```python
from build123d import *

# Parameters (mm, degrees)
BOSS_EXTRUDE1_DEPTH            = 34
BOSS_EXTRUDE1_2_DEPTH          = 34
SKETCH5_W                      = 38.2
SKETCH5_H                      = 34
BOSS_EXTRUDE2_DEPTH            = 16
BOSS_EXTRUDE7_REACH            = 77.954
SKETCH12_W                     = 2
SKETCH12_H                     = 5
BOSS_EXTRUDE8_REACH            = 79.938
SKETCH13_W                     = 2
SKETCH13_H                     = 5
CUT_EXTRUDE1_START             = 2
SKETCH6_W                      = 4
SKETCH6_H                      = 5
CUT_EXTRUDE1_DEPTH             = 14
SKETCH7_W                      = 49
SKETCH7_H                      = 44
BOSS_EXTRUDE3_DEPTH            = 2
SKETCH8_W                      = 10
SKETCH8_H                      = 5
SKETCH8_W_2                    = 2
BOSS_EXTRUDE5_DEPTH            = 45
CUT_EXTRUDE2_REACH             = 97.297
SKETCH9_W                      = 6
SKETCH9_H                      = 44
CUT_EXTRUDE2_DIRECTION_2_REACH = 97.297
SKETCH10_W                     = 23
SKETCH10_H                     = 24
CUT_EXTRUDE3_DEPTH             = 16
SKETCH11_W                     = 2
SKETCH11_H                     = 5
BOSS_EXTRUDE6_DEPTH            = 37
SKETCH14_W                     = 5
SKETCH14_H                     = 34
CUT_EXTRUDE4_DEPTH             = 5.320889


with BuildPart() as part:
    # Sketch4 → Boss-Extrude1 (new body)
    with BuildSketch(Plane.XY):
        Polygon((0, 0), (-14.095389312, 0), (0, 5.13030215), align=None)
    extrude(amount=BOSS_EXTRUDE1_DEPTH)



with BuildPart() as body_2:
    # Sketch4 → Boss-Extrude1 2 (new body)
    with BuildSketch(Plane.XY):
        Polygon((52.295389312, 0), (38.2, 5.13030215), (38.2, 0), align=None)
    extrude(amount=BOSS_EXTRUDE1_2_DEPTH)


with BuildPart() as part_1:
    add(part.part)

    add(body_2.part)  # Boss-Extrude2 merges body 2
    # Sketch5 → Boss-Extrude2 (add)
    with BuildSketch(Plane(origin=(0, 0, 0), x_dir=(1, 0, 0), z_dir=(0, 1, 0))):
        with Locations((19.1, -17)):
            Rectangle(SKETCH5_W, SKETCH5_H)
    extrude(amount=BOSS_EXTRUDE2_DEPTH)

    # Boss-Extrude7: up to this plane
    boss_extrude7_end = Plane(origin=(0, 16, 0), z_dir=(1, 0, 0))
    # Sketch12 → Boss-Extrude7 (add, up to the surface)
    with BuildSketch(Plane(origin=(-12.446541984, -4.530170802, 0), x_dir=(0, 0, -1), z_dir=(0.9396926207859105, 0.3420201433256627, 0)), mode=Mode.PRIVATE) as boss_extrude7_sk1:
        with Locations((-1, 7.320907073)):
            Rectangle(SKETCH12_W, SKETCH12_H)
    boss_extrude7_tool1 = split(extrude(boss_extrude7_sk1.sketch, amount=BOSS_EXTRUDE7_REACH, mode=Mode.PRIVATE), bisect_by=boss_extrude7_end, keep=Keep.BOTH, mode=Mode.PRIVATE)
    add(boss_extrude7_tool1.solids().sort_by_distance((-14.95044, 2.349232, 1))[0])
    # Sketch12 → Boss-Extrude7 (add, up to the surface)
    with BuildSketch(Plane(origin=(-12.446541984, -4.530170802, 0), x_dir=(0, 0, -1), z_dir=(0.9396926207859105, 0.3420201433256627, 0)), mode=Mode.PRIVATE) as boss_extrude7_sk2:
        with Locations((-33, 7.320907073)):
            Rectangle(SKETCH12_W, SKETCH12_H)
    boss_extrude7_tool2 = split(extrude(boss_extrude7_sk2.sketch, amount=BOSS_EXTRUDE7_REACH, mode=Mode.PRIVATE), bisect_by=boss_extrude7_end, keep=Keep.BOTH, mode=Mode.PRIVATE)
    add(boss_extrude7_tool2.solids().sort_by_distance((-14.95044, 2.349232, 33))[0])

    # Boss-Extrude8: up to this plane
    boss_extrude8_end = Plane(origin=(38.2, 16, 0), z_dir=(-1, 0, 0))
    # Sketch13 → Boss-Extrude8 (add, up to the surface)
    with BuildSketch(Plane(origin=(46.177990847, -16.807414147, 0), x_dir=(0, 0, -1), z_dir=(0.9396926207859105, -0.3420201433256628, 0)), mode=Mode.PRIVATE) as boss_extrude8_sk1:
        with Locations((-33, 20.386076548)):
            Rectangle(SKETCH13_W, SKETCH13_H)
    boss_extrude8_tool1 = split(extrude(boss_extrude8_sk1.sketch, amount=-BOSS_EXTRUDE8_REACH, mode=Mode.PRIVATE), bisect_by=boss_extrude8_end, keep=Keep.BOTH, mode=Mode.PRIVATE)
    add(boss_extrude8_tool1.solids().sort_by_distance((53.15044, 2.349232, 33))[0])
    # Sketch13 → Boss-Extrude8 (add, up to the surface)
    with BuildSketch(Plane(origin=(46.177990847, -16.807414147, 0), x_dir=(0, 0, -1), z_dir=(0.9396926207859105, -0.3420201433256628, 0)), mode=Mode.PRIVATE) as boss_extrude8_sk2:
        with Locations((-1, 20.386076548)):
            Rectangle(SKETCH13_W, SKETCH13_H)
    boss_extrude8_tool2 = split(extrude(boss_extrude8_sk2.sketch, amount=-BOSS_EXTRUDE8_REACH, mode=Mode.PRIVATE), bisect_by=boss_extrude8_end, keep=Keep.BOTH, mode=Mode.PRIVATE)
    add(boss_extrude8_tool2.solids().sort_by_distance((53.15044, 2.349232, 1))[0])

    # Sketch6 → Cut-Extrude1 (cut)
    with BuildSketch(Plane(origin=(0, 0, 0), x_dir=(1, 0, 0), z_dir=(0, 1, 0)).offset(CUT_EXTRUDE1_START)):
        with Locations((12.7, -31.5)):
            Rectangle(SKETCH6_W, SKETCH6_H)
        with Locations((25.5, -2.5)):
            Rectangle(SKETCH6_W, SKETCH6_H)
    extrude(amount=CUT_EXTRUDE1_DEPTH, mode=Mode.SUBTRACT)

    # Sketch7 → Boss-Extrude3 (add)
    with BuildSketch(Plane(origin=(0, 0, 0), x_dir=(1, 0, 0), z_dir=(0, 1, 0))):
        with Locations((22.5, -56)):
            Rectangle(SKETCH7_W, SKETCH7_H)
    extrude(amount=BOSS_EXTRUDE3_DEPTH)

    # Sketch8 → Boss-Extrude5 (add)
    with BuildSketch(Plane.XY.offset(78)):
        with Locations((42, 4.5)):
            Rectangle(SKETCH8_W, SKETCH8_H)
        with Locations((-1, 4.5)):
            Rectangle(SKETCH8_W_2, SKETCH8_H)
    extrude(amount=-BOSS_EXTRUDE5_DEPTH)

    # Cut-Extrude2: up to this face of the body (flat: up to its plane)
    cut_extrude2_end = Plane(part_1.part.faces().sort_by_distance((18.42961165, 2, 55.702669903))[0])
    # Sketch9 → Cut-Extrude2 (cut, up to the picked face)
    with BuildSketch(Plane(origin=(0, 7, 0), x_dir=(1, 0, 0), z_dir=(0, 1, 0)), mode=Mode.PRIVATE) as cut_extrude2_sk1:
        with Locations((42, -56)):
            Rectangle(SKETCH9_W, SKETCH9_H)
    cut_extrude2_tool1 = split(extrude(cut_extrude2_sk1.sketch, amount=-CUT_EXTRUDE2_REACH, mode=Mode.PRIVATE), bisect_by=cut_extrude2_end, keep=Keep.BOTH, mode=Mode.PRIVATE)
    add(cut_extrude2_tool1.solids().sort_by(Axis((42, 7, 56), (0, -1, 0)))[0], mode=Mode.SUBTRACT)

    # Cut-Extrude2 direction 2: up to this face of the body (flat: up to its plane)
    cut_extrude2_direction_2_end = Plane(part_1.part.faces().sort_by_distance((46.102745014, 7.574827058, 33))[0])
    # Sketch9 → Cut-Extrude2 direction 2 (cut, up to the picked face)
    with BuildSketch(Plane(origin=(0, 7, 0), x_dir=(1, 0, 0), z_dir=(0, 1, 0)), mode=Mode.PRIVATE) as cut_extrude2_direction_2_sk1:
        with Locations((42, -56)):
            Rectangle(SKETCH9_W, SKETCH9_H)
    cut_extrude2_direction_2_tool1 = split(extrude(cut_extrude2_direction_2_sk1.sketch, amount=CUT_EXTRUDE2_DIRECTION_2_REACH, mode=Mode.PRIVATE), bisect_by=cut_extrude2_direction_2_end, keep=Keep.BOTH, mode=Mode.PRIVATE)
    add(cut_extrude2_direction_2_tool1.solids().sort_by(Axis((42, 7, 56), (0, 1, 0)))[0], mode=Mode.SUBTRACT)

    # Sketch10 → Cut-Extrude3 (cut)
    with BuildSketch(Plane(origin=(0, 16, 0), x_dir=(1, 0, 0), z_dir=(0, 1, 0))):
        with Locations((19.1, -17)):
            Rectangle(SKETCH10_W, SKETCH10_H)
    extrude(amount=-CUT_EXTRUDE3_DEPTH, mode=Mode.SUBTRACT)

    # Sketch11 → Boss-Extrude6 (add)
    with BuildSketch(Plane(origin=(0, 0, 0), x_dir=(0, 0, -1), z_dir=(1, 0, 0))):
        with Locations((-77, 4.5)):
            Rectangle(SKETCH11_W, SKETCH11_H)
    extrude(amount=BOSS_EXTRUDE6_DEPTH)

    # Sketch14 → Cut-Extrude4 (cut)
    with BuildSketch(Plane(origin=(0, 0, 0), x_dir=(1, 0, 0), z_dir=(0, 1, 0))):
        with Locations((-16.595389312, -17)):
            Rectangle(SKETCH14_W, SKETCH14_H)
        with Locations((54.795389312, -17)):
            Rectangle(SKETCH14_W, SKETCH14_H)
    extrude(amount=CUT_EXTRUDE4_DEPTH, mode=Mode.SUBTRACT)


solid = part_1.part
```
Input: part model. Units: mm. Frame: model coordinates. A direction names the side the tool comes from. Round coordinates to 2 decimals unless told otherwise and drop trailing zeros. Loops run counter-clockwise (first coordinate to the right, second up) from the corner with the lowest first, then second, coordinate; pieces in that order, holes last. Notation, with made-up numbers: (53.25, 25) -> (72.25, 25) arc R24 ccw to (72.25, 47) -> close; hole circle Ø8 at (-19.5, -29). An arc over 180 degrees is marked (long way). Use one line per item in the form item = value. Start each with the question number.
Item 1: Mould query, pull axis X, two halves, no side actions, for faces 4 (the face through (-0.2, 7.3, 34)), 5 (the face through (6, 16, 13)), 6 (the face through (-7.15, 7.85, 33.01)). Classes: pulls with the +X half, pulls with the -X half, needs draft (parallel to the pull), parting line crosses it, or undercut.
Item 2: Material intervals for L1, parallel to X at y = 3.5, z = 60.5; L2, parallel to Z at x = 26, y = 3.5; L3, parallel to Z at x = 48, y = 5.25, sorted ascending. Write a range as from..to.
Item 3: Section query B-B on y = 13. Return the cut outline in (x, z), then the cut area to 3 significant figures.
Item 4: Section query D-D on z = 61.5. Return the cut outline in (x, y), then the cut area to 3 significant figures.
Item 5: Contact query for flat-ended pins moving along their axis: pin 1 Ø12 at (x, z) = (19, 38.5) entering from +Y; pin 2 Ø5.5 at (y, z) = (4, 57) entering from -X; pin 3 Ø18.5 at (x, z) = (14, 53.5) entering from +Y; pin 4 Ø5 at (y, z) = (10.5, 15) entering from -X. Output: stop coordinate, or through.
Item 6: Section query C-C on z = 7. Return the cut outline in (x, y), then the cut area to 3 significant figures.
Item 7: Section query A-A on x = 22. Return the cut outline in (y, z).
Item 8: Set-up query: faces 1 (the face through (45, 5, 32)), 2 (the face through (0, 10, 17)), 3 (the face through (18, 7, 77)). Return all of +Z, -Z, +X, -X, +Y, -Y with unobstructed straight access to the full face (end or side cutting, diameter ignored); none if empty.
Ans:
q1.face_4 = undercut
q1.face_5 = needs draft
q1.face_6 = pulls with the -X half
q2.L1 = -2..0, 37..39, 45..47
q2.L2 = 29..34, 76..78
q2.L3 = 0..2, 32..34
q3.outline = (0, 0) -> (23.5, 0) -> (23.5, 5) -> (7.6, 5) -> (7.6, 29) -> (10.7, 29) -> (10.7, 34) -> (0, 34) -> close; (14.7, 29) -> (30.6, 29) -> (30.6, 5) -> (27.5, 5) -> (27.5, 0) -> (38.2, 0) -> (38.2, 34) -> (14.7, 34) -> close
q3.area = 707 mm^2
q4.outline = (-2, 0) -> (47, 0) -> (47, 7) -> (45, 7) -> (45, 2) -> (39, 2) -> (39, 7) -> (37, 7) -> (37, 2) -> (0, 2) -> (0, 7) -> (-2, 7) -> close
q4.area = 128 mm^2
q5.pin_1 = 16
q5.pin_2 = -2
q5.pin_3 = 2
q5.pin_4 = 0
q6.outline = (-14.1, 0) -> (7.6, 0) -> (7.6, 16) -> (0, 16) -> (0, 5.13) -> close; (30.6, 0) -> (52.3, 0) -> (38.2, 5.13) -> (38.2, 16) -> (30.6, 16) -> close
q6.area = 316 mm^2
q7.outline = (0, 0) -> (16, 0) -> (16, 5) -> (0, 5) -> close; (0, 29) -> (16, 29) -> (16, 34) -> (2, 34) -> (2, 76) -> (7, 76) -> (7, 78) -> (0, 78) -> close
q8.face_1 = +X, +Y
q8.face_2 = -X, +Y
q8.face_3 = +Z, +X, -X, +Y
